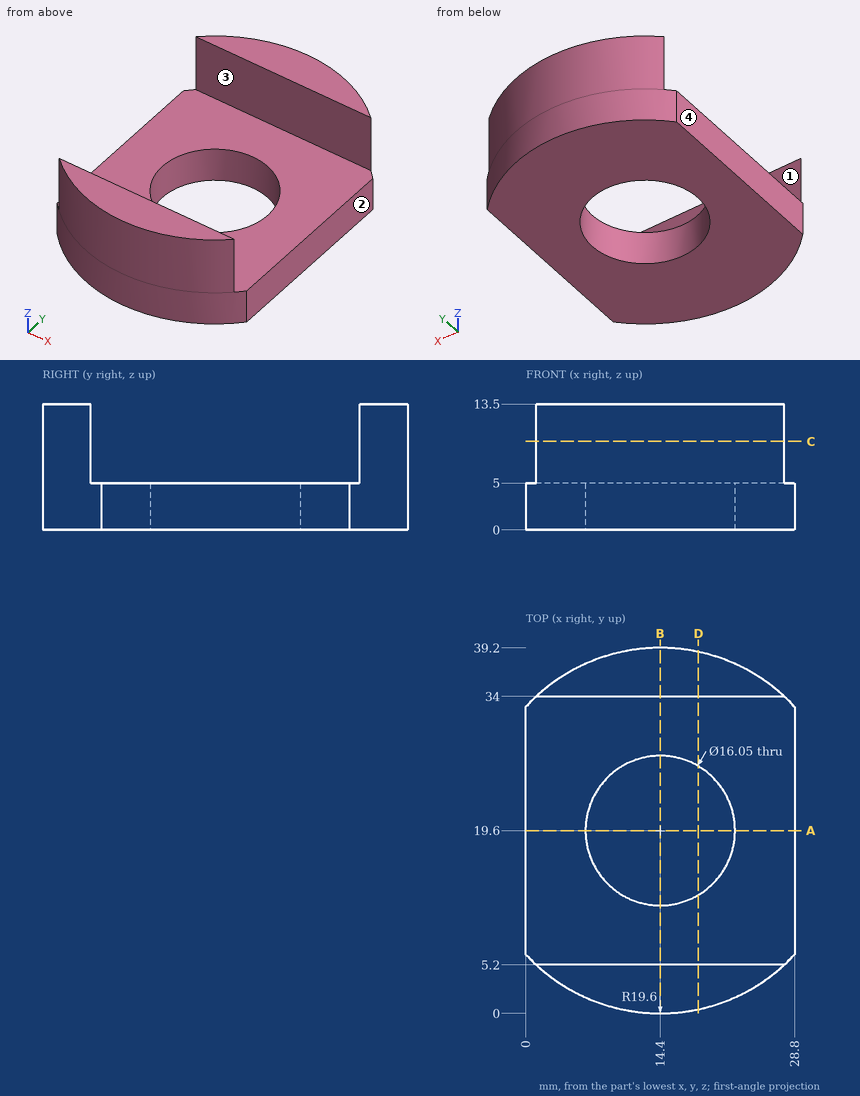
For this review, use the dimensioned drawing (mm, ordinates from the lowest corner) and the shaded views. A direction names the side the tool comes from. Coordinates: 2 decimals unless noted, no trailing zeros. Order: outer loops, then holes, each group sorted by start corner. A loop starts at its lowest first (then second) coordinate and runs counter-clockwise, first axis right, second up. Notation, with made-up numbers: (36.5, 63.5) - (81.5, 63.5) arc R21 ccw to (81.5, 71.5) - close; hole circle Ø5 at (-12, -2.75). An arc over 180 degrees is marked (long way). Answer in a Markdown table with one row per item.
(1) Consider section C-C on z = 9.5. State the section outline as (x, y) points.
Checked values:
| item | result |
|---|---|
| outline | (1.1, 5.2) arc R19.6 ccw to (27.7, 5.2) - close; (1.1, 34) - (27.7, 34) arc R19.6 ccw to start |
(2) Wall thickness on line 1 along Z through (x, y) = (4, 12.5); line 2 along Y through (x, z) = (22, 11.5); line 3 along Y through (x, z) = (26.25, 6.5): over which ranges is each line inside the solid? List them lowest first. Write a range as from..to.
Checked values:
| item | result |
|---|---|
| line 1 | 0..5 |
| line 2 | 1.53..5.2, 34..37.67 |
| line 3 | 3.99..5.2, 34..35.21 |
(3) For the marked faces 1 and 2, list the 3-axis set-ups (+Z, -Z, +X, -X, +Y, -Y) from which the entire face can be reached by the end or side of a thin tool; tool diameter is ignored.
Checked values:
| item | result |
|---|---|
| face 1 | +Z, +X, -X |
| face 2 | +Z, -Z, +X, +Y, -Y |
(4) Clearance check with flat-ended pins moving along their axes: pin 1 (4 mm diameter, centred on x = 24, y = 20.5, fed in from +Z); pin 2 (8 mm diameter, centred on x = 9.5, z = 6.5, fed in from -Y); pin 3 (2.5 mm diameter, centred on x = 10.5, z = 9.5, fed in from -Y). State where each tip first meets the part, or that it passes through.
Checked values:
| item | result |
|---|---|
| pin 1 | z = 5 |
| pin 2 | y = 0.02 |
| pin 3 | y = 0.18 |
(5) Consider section A-A on y = 19.6. State the section outline as (x, z) points (3 decimals).
Checked values:
| item | result |
|---|---|
| outline | (0, 0) - (6.375, 0) - (6.375, 5) - (0, 5) - close; (22.425, 0) - (28.8, 0) - (28.8, 5) - (22.425, 5) - close |
(6) The part is to be moulded in two halves that separate along Y. For the marked faces 3 and 4, say which applies: released by +Y, released by -Y, zero draft, split by the parting line, or undercut.
Checked values:
| item | result |
|---|---|
| face 3 | undercut |
| face 4 | zero draft |
(7) Consider section B-B on x = 14.4. State the section outline as (y, z) points (3 decimals).
Checked values:
| item | result |
|---|---|
| outline | (0, 0) - (11.575, 0) - (11.575, 5) - (5.2, 5) - (5.2, 13.5) - (0, 13.5) - close; (27.625, 0) - (39.2, 0) - (39.2, 13.5) - (34, 13.5) - (34, 5) - (27.625, 5) - close |
(8) Consider section D-D on x = 18.5. State the section outline as (y, z) points.
Checked values:
| item | result |
|---|---|
| outline | (0.43, 0) - (12.7, 0) - (12.7, 5) - (5.2, 5) - (5.2, 13.5) - (0.43, 13.5) - close; (26.5, 0) - (38.77, 0) - (38.77, 13.5) - (34, 13.5) - (34, 5) - (26.5, 5) - close |
